from build123d import *

# Parameters (mm, degrees)
SKETCH1_W                      = 20
SKETCH1_H                      = 5
EXTRUDE1_DEPTH                 = 6.2
SKETCH2_W                      = 10.51
SKETCH2_H                      = 5
EXTRUDE3_DEPTH                 = 1.5
SKETCH3_W                      = 6.51
SKETCH3_H                      = 5
EXTRUDE4_DEPTH                 = 1.63
CBORE_FOR_M2_SHCS1_D           = 2.4
CBORE_FOR_M2_SHCS1_CBORE_D     = 4.4
CBORE_FOR_M2_SHCS1_CBORE_DEPTH = 2
LPATTERN1_COUNT                = 2
LPATTERN1_PITCH                = 15
M2X0_4_TAPPED_HOLE1_D          = 1.6
LPATTERN3_COUNT                = 2
LPATTERN3_PITCH                = 3


with BuildPart() as part:
    # Sketch1 → Extrude1 (new body)
    with BuildSketch(Plane(origin=(0, 0, 0), x_dir=(1, 0, 0), z_dir=(0, 1, 0))):
        Rectangle(SKETCH1_W, SKETCH1_H)
    extrude(amount=EXTRUDE1_DEPTH)

    # Sketch2 → Extrude3 (cut)
    with BuildSketch(Plane(origin=(0, 6.2, 0), x_dir=(1, 0, 0), z_dir=(0, 1, 0))):
        Rectangle(SKETCH2_W, SKETCH2_H)
    extrude(amount=-EXTRUDE3_DEPTH, mode=Mode.SUBTRACT)

    # Sketch3 → Extrude4 (cut)
    with BuildSketch(Plane(origin=(0, 4.7, 0), x_dir=(1, 0, 0), z_dir=(0, 1, 0))):
        Rectangle(SKETCH3_W, SKETCH3_H)
    extrude(amount=-EXTRUDE4_DEPTH, mode=Mode.SUBTRACT)

    # CBORE for M2 SHCS1 (through all)
    with Locations(Plane(origin=(-7.5, 0, 0), x_dir=(0, 0, -1), z_dir=(0, -1, 0))):
        with Locations((0, 0)):
            cbore_for_m2_shcs1 = CounterBoreHole(CBORE_FOR_M2_SHCS1_D / 2, CBORE_FOR_M2_SHCS1_CBORE_D / 2, CBORE_FOR_M2_SHCS1_CBORE_DEPTH)

    # LPattern1: CBORE for M2 SHCS1 ×2
    with Locations(*[(i * LPATTERN1_PITCH, 0, 0) for i in range(1, LPATTERN1_COUNT)]):
        add(cbore_for_m2_shcs1, mode=Mode.SUBTRACT)

    # M2x0.4 Tapped Hole1 (through all)
    with Locations(Plane(origin=(-1.5, 0, 0), x_dir=(0, 0, -1), z_dir=(0, -1, 0))):
        with Locations((0, 0)):
            m2x0_4_tapped_hole1 = Hole(M2X0_4_TAPPED_HOLE1_D / 2)

    # LPattern3: M2x0.4 Tapped Hole1 ×2
    with Locations(*[(i * LPATTERN3_PITCH, 0, 0) for i in range(1, LPATTERN3_COUNT)]):
        add(m2x0_4_tapped_hole1, mode=Mode.SUBTRACT)


solid = part.part
Geometry: final body of the model. Coordinates: model frame, mm. A direction names the side the tool comes from. Give positions to 0.01 mm unless a question says otherwise; leave off trailing zeros. Loops run counter-clockwise (first coordinate to the right, second up) from the corner with the lowest first, then second, coordinate; pieces in that order, holes last. Notation, with made-up numbers: (-9, 87) -> (18, 87) arc R19 cw to (18, 113) -> close; hole circle Ø8 at (-20.5, -37.5). An arc over 180 degrees is marked (long way). Put each result on its own line as item: value.
1. Cut plane A-A (y = 5). Return the cut outline in (x, z) (3 decimals).
Taken from the geometry:
outline: (-10, -2.5) -> (-5.255, -2.5) -> (-5.255, 2.5) -> (-10, 2.5) -> close; (5.255, -2.5) -> (10, -2.5) -> (10, 2.5) -> (5.255, 2.5) -> close; hole circle Ø2.4 at (-7.5, 0); hole circle Ø2.4 at (7.5, 0)
2. Cut plane B-B (x = 1.5). Return the cut outline in (y, z), plus the area to 3 significant figures.
Taken from the geometry:
outline: (0, -2.5) -> (3.07, -2.5) -> (3.07, -0.8) -> (0, -0.8) -> close; (0, 0.8) -> (3.07, 0.8) -> (3.07, 2.5) -> (0, 2.5) -> close
area: 10.4 mm2
3. Set-up query: faces 4 (the cylindrical face through (9.355, 0.986, -1.183)), 5 (the flat face through (0, 0, 0)), 6 (the flat face through (0, 3.07, 0)). Return all of +Z, -Z, +X, -X, +Y, -Y with unobstructed straight access to the full face (end or side cutting, diameter ignored); none if empty.
Taken from the geometry:
face 4: -Y
face 5: +Z, -Z, +X, -X, -Y
face 6: +Z, -Z, +Y
4. Pin query (flat end, axial travel): P1, Ø2, axis at x = -4, z = -0.5, coming from the +Y side; P2, Ø1.6, axis at x = 4.5, z = 1, coming from the +Y side; P3, Ø2, axis at x = 8, z = 0, coming from the -Y side; P4, Ø2.5, axis at x = -1.5, z = 0.5, coming from the +Y side. Return the tip coordinate at first contact, or that it passes through.
Taken from the geometry:
P1: stops at y = 4.7
P2: stops at y = 6.2
P3: stops at y = 2
P4: stops at y = 3.07
5. Ray query, line 1 along X through (y, z) = (3.25, 0) (3 decimals); line 2 along X through (y, z) = (5.25, -1.65) (3 decimals); line 3 along X through (y, z) = (1.3, 0). Return the intervals inside material, ascending. Write a range as [from, to].
Taken from the geometry:
line 1: x = [-10, -8.7], [-6.3, -3.255], [3.255, 6.3], [8.7, 10]
line 2: x = [-10, -5.255], [5.255, 10]
line 3: x = [-10, -9.7], [-5.3, -2.3], [-0.7, 0.7], [2.3, 5.3], [9.7, 10]
6. Pull-direction query (X, two-part tool) for faces 1 (the flat face through (-9, 2, 0)), 2 (the flat face through (10, 3, 0)), 3 (the flat face through (9, 6.2, -1)); classes: released by +X, released by -X, zero draft, split by the parting line, or undercut.
Taken from the geometry:
face 1: undercut
face 2: released by +X
face 3: zero draft
7. Cut plane C-C (y = 1.75). Return the cut outline in (x, z).
Taken from the geometry:
outline: (-10, -2.5) -> (10, -2.5) -> (10, 2.5) -> (-10, 2.5) -> close; hole circle Ø4.4 at (-7.5, 0); hole circle Ø1.6 at (-1.5, 0); hole circle Ø1.6 at (1.5, 0); hole circle Ø4.4 at (7.5, 0)
8. Cut plane D-D (x = 7.5). Return the cut outline in (y, z), plus the area to 3 significant figures.
Taken from the geometry:
outline: (0, -2.5) -> (6.2, -2.5) -> (6.2, -1.2) -> (2, -1.2) -> (2, -2.2) -> (0, -2.2) -> close; (0, 2.2) -> (2, 2.2) -> (2, 1.2) -> (6.2, 1.2) -> (6.2, 2.5) -> (0, 2.5) -> close
area: 12.1 mm2
